Design review of the part built by this model. Coordinates are the model's own, in mm. Face numbers are marked on the shaded views. A direction names the side the tool comes from. Give positions to 0.01 mm unless a question says otherwise; leave off trailing zeros. Write each loop counter-clockwise with the first axis right and the second up, starting at its lowest first coordinate (ties: lowest second). Pieces come first, ordered by that corner, then holes. Notation, with made-up numbers: (66.5, -30.75) -> (111.5, -30.75) arc R7 cw to (111.5, -22.75) -> close; hole circle Ø3 at (-39, 35). An arc over 180 degrees is marked (long way). Answer as a JSON object with one key per item and string values.
```python
from build123d import *

# Parameters (mm, degrees)
SKETCH1_R                                     = 87.5
SKETCH1_R_2                                   = 82.5
BOSS_EXTRUDE1_DEPTH                           = 50
CUT_EXTRUDE1_DEPTH                            = 134.46347815
BOSS_EXTRUDE2_REACH                           = 201.927
BOSS_EXTRUDE2_END_RADIUS                      = 82.5
MIRROR1_AT_THE_SECOND_PLANE_COPY_1_DEPTH      = 134.46347815
MIRROR1_AT_THE_SECOND_PLANE_COPY_2_REACH      = 201.927
MIRROR1_AT_THE_SECOND_PLANE_COPY_2_END_RADIUS = 82.5
SKETCH4_W                                     = 75
SKETCH4_H                                     = 150.506250548
CUT_EXTRUDE2_DEPTH                            = 134.463478319


with BuildPart() as part:
    # Sketch1 → Boss-Extrude1 (new body)
    with BuildSketch(Plane.XY):
        Circle(SKETCH1_R)
        Circle(SKETCH1_R_2, mode=Mode.SUBTRACT)
    extrude(amount=BOSS_EXTRUDE1_DEPTH)

    # Sketch3 → Cut-Extrude1 (cut, through all)
    with BuildSketch(Plane(origin=(0, 0, 0), x_dir=(0, 0, 1), z_dir=(-0.7660444431189792, 0.6427876096865379, 0))):
        with BuildLine():
            Line((16, 28), (-21.315886337, 28))
            Line((-21.315886337, 28), (-21.315886337, -28))
            Line((-21.315886337, -28), (16, -28))
            ThreePointArc((16, -28), (44, 0), (16, 28))
        make_face()
    cut_extrude1 = extrude(amount=CUT_EXTRUDE1_DEPTH, mode=Mode.SUBTRACT)

    # Boss-Extrude2: up to this cylinder (the profile starts inside it)
    boss_extrude2_end = Plane(origin=(0, 0, 8), z_dir=(0, 0, -1)) * Cylinder(BOSS_EXTRUDE2_END_RADIUS, 569.854, mode=Mode.PRIVATE)
    # Sketch5 → Boss-Extrude2 (add, up to the surface)
    with BuildSketch(Plane(origin=(-53.623111018, 44.995132678, 0), x_dir=(0, 0, 1), z_dir=(-0.7660444431189792, 0.6427876096865379, 0)), mode=Mode.PRIVATE) as boss_extrude2_sk1:
        with BuildLine():
            Line((0, -28), (16, -28))
            ThreePointArc((16, -28), (44, 0), (16, 28))
            Line((16, 28), (0, 28))
            Line((0, 28), (0, 30))
            Line((0, 30), (16, 30))
            ThreePointArc((16, 30), (46, 0), (16, -30))
            Line((16, -30), (0, -30))
            Line((0, -30), (0, -28))
        make_face()
    boss_extrude2_tool1 = extrude(boss_extrude2_sk1.sketch, amount=BOSS_EXTRUDE2_REACH, mode=Mode.PRIVATE) & boss_extrude2_end
    boss_extrude2 = boss_extrude2_tool1.solids().sort_by_distance((-72.420765, 22.592961, 8))[0]
    add(boss_extrude2)

    # Mirror1: Cut-Extrude1, Boss-Extrude2 across plane
    add(cut_extrude1.mirror(Plane(origin=(0, 0, 0), x_dir=(0, 0, 1), z_dir=(1, 0, 0))), mode=Mode.SUBTRACT)
    add(boss_extrude2.mirror(Plane(origin=(0, 0, 0), x_dir=(0, 0, 1), z_dir=(1, 0, 0))))

    # Mirror1 at the second plane: Cut-Extrude1, Boss-Extrude2 across plane
    add(cut_extrude1.mirror(Plane.ZX), mode=Mode.SUBTRACT)
    add(boss_extrude2.mirror(Plane.ZX))

    # Mirror1 at the second plane copy 1 sketc → Mirror1 at the second plane copy 1 (cut, through all)
    with BuildSketch(Plane(origin=(0, 0, 0), x_dir=(0, 0, 1), z_dir=(0.7660444431189792, -0.6427876096865379, 0))):
        with BuildLine():
            Line((16, 28), (-21.315886337, 28))
            Line((-21.315886337, 28), (-21.315886337, -28))
            Line((-21.315886337, -28), (16, -28))
            ThreePointArc((16, -28), (44, 0), (16, 28))
        make_face()
    extrude(amount=MIRROR1_AT_THE_SECOND_PLANE_COPY_1_DEPTH, mode=Mode.SUBTRACT)

    # Mirror1 at the second plane copy 2: up to this cylinder (the profile starts inside it)
    mirror1_at_the_second_plane_copy_2_end = Plane(origin=(0, 0, 8), z_dir=(0, 0, -1)) * Cylinder(MIRROR1_AT_THE_SECOND_PLANE_COPY_2_END_RADIUS, 569.854, mode=Mode.PRIVATE)
    # Mirror1 at the second plane copy 2 sketc → Mirror1 at the second plane copy 2 (add, up to the surface)
    with BuildSketch(Plane(origin=(53.623111018, -44.995132678, 0), x_dir=(0, 0, 1), z_dir=(0.7660444431189792, -0.6427876096865379, 0)), mode=Mode.PRIVATE) as mirror1_at_the_second_plane_copy_2_sk1:
        with BuildLine():
            Line((0, -28), (16, -28))
            ThreePointArc((16, -28), (44, 0), (16, 28))
            Line((16, 28), (0, 28))
            Line((0, 28), (0, 30))
            Line((0, 30), (16, 30))
            ThreePointArc((16, 30), (46, 0), (16, -30))
            Line((16, -30), (0, -30))
            Line((0, -30), (0, -28))
        make_face()
    mirror1_at_the_second_plane_copy_2_tool1 = extrude(mirror1_at_the_second_plane_copy_2_sk1.sketch, amount=MIRROR1_AT_THE_SECOND_PLANE_COPY_2_REACH, mode=Mode.PRIVATE) & mirror1_at_the_second_plane_copy_2_end
    add(mirror1_at_the_second_plane_copy_2_tool1.solids().sort_by_distance((-72.420765, 22.592961, 8))[0])

    # Sketch4 → Cut-Extrude2 (cut, through all)
    with BuildSketch(Plane.XY.offset(50)):
        with Locations((0, 75.253125274)):
            Rectangle(SKETCH4_W, SKETCH4_H)
    extrude(amount=-CUT_EXTRUDE2_DEPTH, mode=Mode.SUBTRACT)


solid = part.part
```
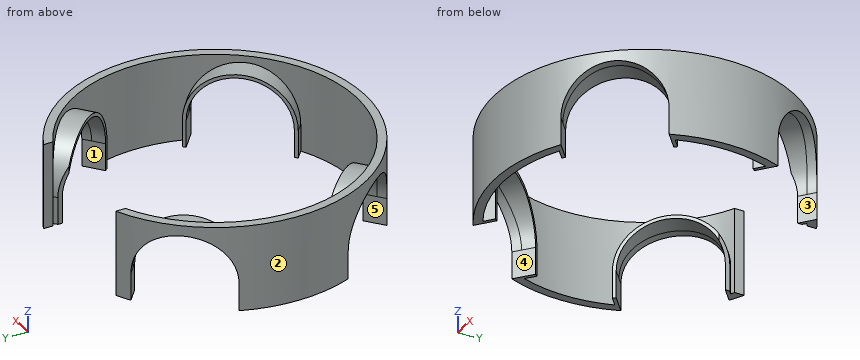
(1) We need section B-B, the plane z = 13. Give the number of separate pieces and of enclosed holes in the cut face, then the cut area to 3 significant figures.
Here are the results:
{"separate pieces": "5", "enclosed holes": "0", "area": "1,240 mm²"}
(2) For the marked faces 1 and 2, list the 3-axis set-ups (+Z, -Z, +X, -X, +Y, -Y) from which the entire face can be reached by the end or side of a thin tool; tool diameter is ignored.
Here are the results:
{"face 1": "-Z, +Y", "face 2": "+Z, -Z"}
(3) We need section C-C, the plane x = 0. State the section outline as (y, z) points.
Here are the results:
{"outline": "(-87.5, 0) -> (-82.5, 0) -> (-82.5, 50) -> (-87.5, 50) -> close"}
(4) For line 1 along X through (y, z) = (0, 11.5); line 2 along X through (y, z) = (27, 25); line 3 along Y through (x, z) = (46, 36), list the stretches that pass through material, from the lowest coordinate up.
Here are the results:
{"line 1": "x = -87.5 to -82.5, 82.5 to 87.5", "line 2": "x = -83.23 to -77.96, -76.7 to -73.43, 73.43 to 76.7, 77.96 to 83.23", "line 3": "y = -74.43 to -68.49, -67.79 to -64.18, 64.18 to 67.79, 68.49 to 74.43"}
(5) The part is to be moulded in two halves that separate along X. For the marked faces 3, 4 and 5, say which applies: +X half, -X half, draft (parallel to the pull), parting line (faces both ways), or undercut.
Here are the results:
{"face 3": "+X half", "face 4": "undercut", "face 5": "-X half"}
(6) We need section A-A, the plane y = 0. State the section outline as (x, z) points, then the cut area to 3 significant figures.
Here are the results:
{"outline": "(-87.5, 0) -> (-82.5, 0) -> (-82.5, 50) -> (-87.5, 50) -> close; (82.5, 0) -> (87.5, 0) -> (87.5, 50) -> (82.5, 50) -> close", "area": "500 mm²"}
(7) Clearance check with flat-ended pins moving along their axes: pin 1 (3 mm diameter, centred on y = -26, z = 39.5, fed in from -X); pin 2 (1.5 mm diameter, centred on y = -70.5, z = 7.5, fed in from -X); pin 3 (1 mm diameter, centred on y = -1, z = 9.5, fed in from +X); pin 4 (1.9 mm diameter, centred on y = 66.5, z = 15.5, fed in from +X). State where each tip first meets the part, or that it passes through.
Here are the results:
{"pin 1": "stops at x = -84", "pin 2": "stops at x = -41.35", "pin 3": "stops at x = 87.5", "pin 4": "passes through"}
